Here's how the part is built. I have some questions about the finished solid (model axes, mm). A direction names the side the tool comes from. Give positions to 0.01 mm unless a question says otherwise; leave off trailing zeros. Loops run counter-clockwise (first coordinate to the right, second up) from the corner with the lowest first, then second, coordinate; pieces in that order, holes last. Notation, with made-up numbers: (82, 38) - (124, 38) arc R31 cw to (124, 68) - close; hole circle Ø9 at (25, -21). An arc over 180 degrees is marked (long way). Use one line per item in the form item = value.
from build123d import *

# Parameters (mm, degrees)
F1_DEPTH = 30
F2_SIZE2 = 5.08
F2_SIZE  = 5.08


with BuildPart() as f1:
    # F0 (on Top) → F1 (new body)
    with BuildSketch(Plane.XY):
        Polygon((-48.136686, -28.986598), (-48.904475, -7), (101.095525, -7), (101.095525, 20), (86.173893, 37.782908), (83.239773, 35.320889), (96.095525, 20), (96.095525, 0), (46.095525, 0), (46.095525, 20), (31.173893, 37.782908), (28.23475, 35.316674), (41.095525, 19.9898), (41.095525, 0), (-8.904475, 0), (-8.904475, 19.9898), (-23.834665, 37.782908), (-26.773808, 35.316674), (-13.913034, 19.9898), (-13.913034, 0), (-56.153187, 0), (-55.132422, -29.230895), align=None)
    extrude(amount=F1_DEPTH)

    # F2
    f2_edges = [f1.edges().sort_by_distance(p)[0] for p in [
        (-25.304237, 36.549791, 30),
        (-25.304237, 36.549791, 0),
        (29.704322, 36.549791, 0),
        (29.704322, 36.549791, 30),
        (84.706833, 36.551899, 30),
        (84.706833, 36.551899, 0),
    ]]
    chamfer(f2_edges, length=F2_SIZE, length2=F2_SIZE2)


solid = f1.part
(1) If we section it at D-D (x = 80.5): List the corners of the cut face in (y, z) for me.
Geometry says:
outline = (-7, 0) - (0, 0) - (0, 30) - (-7, 30) - close
(2) For faces 1 (the flat face through (-13.913, 10, 15)), 2 (the flat face through (34.575, 27.761, 14.79)), 3 (the flat face through (29.725, 36.567, 14.861)), which set-ups out of +Z, -Z, +X, -X, +Y, -Y let a thin tool reach every point of the face, with its end or its side?
Geometry says:
face_1 = +Z, -Z, -X
face_2 = +Z, -Z
face_3 = +Z, -Z, +Y
(3) Thinking about a two-plate mould opening in Y: for faces 4 (the flat face through (71, 0, 15)), 5 (the flat face through (84.73, 36.57, 14.86)), 6 (the flat face through (89.578, 27.768, 14.79)), 7 (the flat face through (101.096, 6, 15)), which applies, pulls with the +Y half, pulls with the -Y half, needs draft (parallel to the pull), parting line crosses it, or undercut?
Geometry says:
face_4 = undercut
face_5 = pulls with the +Y half
face_6 = undercut
face_7 = needs draft
(4) If we section it at B-B (z = 7.5): List the corners of the cut face in (x, y) for me, plus the area to 3 significant figures.
Geometry says:
outline = (-56.15, 0) - (-55.13, -29.23) - (-48.14, -28.99) - (-48.9, -7) - (101.1, -7) - (101.1, 20) - (86.17, 37.78) - (83.24, 35.32) - (96.1, 20) - (96.1, 0) - (46.1, 0) - (46.1, 20) - (31.17, 37.78) - (28.23, 35.32) - (41.1, 19.99) - (41.1, 0) - (-8.9, 0) - (-8.9, 19.99) - (-23.83, 37.78) - (-26.77, 35.32) - (-13.91, 19.99) - (-13.91, 0) - close
area = 1,800 mm²
(5) If we section it at A-A (y = 16.5): List the corners of the cut face in (x, z) for me, plus the area to 3 significant figures.
Geometry says:
outline = (-13.91, 0) - (-8.9, 0) - (-8.9, 30) - (-13.91, 30) - close; (41.1, 0) - (46.1, 0) - (46.1, 30) - (41.1, 30) - close; (96.1, 0) - (101.1, 0) - (101.1, 30) - (96.1, 30) - close
area = 450 mm²
(6) If we section it at C-C (x = 38.5): List the corners of the cut face in (y, z) for me.
Geometry says:
outline = (-7, 0) - (0, 0) - (0, 30) - (-7, 30) - close; (23.08, 0) - (29.05, 0) - (29.05, 30) - (23.08, 30) - close
(7) For P1, Ø9, axis at x = 47, z = 12.5, coming from the -Y side; P2, Ø16, axis at y = 13.5, z = 16, coming from the -X side; P3, Ø10, axis at x = 25.5, z = 23.5, coming from the +Y side, each with a flat end and sliding along its axis, tell me the tip position at first contact or that it passes through.
Geometry says:
P1 = -7
P2 = -15.18
P3 = 37.22
(8) If I drill on probe 1 along X at (y, z) = (10, 22.5); probe 2 along Y at (x, z) = (-47.5, 5); probe 3 along Y at (x, z) = (33, 21.5), over which ranges is the centre line in solid material (lowest first)?
Geometry says:
probe_1 = -13.91 to -8.9, 41.1 to 46.1, 96.1 to 101.1
probe_2 = -7 to 0
probe_3 = -7 to 0, 29.64 to 35.61
